Model file for the job. Use its own axes, mm. A direction names the side the tool comes from. Give positions to 0.01 mm unless a question says otherwise; leave off trailing zeros. Order: outer loops, then holes, each group sorted by start corner. A loop starts at its lowest first (then second) coordinate and runs counter-clockwise, first axis right, second up. Notation, with made-up numbers: (-23, 3.25) -> (16, 3.25) arc R26 cw to (16, 28.25) -> close; hole circle Ø8 at (65, 50.5). An arc over 180 degrees is marked (long way). Use CSV: the item, a comma, the result in double quotes. Start each with the question number.
1. Cut at D-D on x = 240.5. List the corners of the cut face in (y, z).
2. 3-axis set-ups, long thin cutter, end or side, ignore diameter. For faces 5 (the flat face through (238.6, 4.3, 3.2)), 6 (the flat face through (243, -5.677, 9)), 7 (the flat face through (241, 4, 0)): which of +Z, -Z, +X, -X, +Y, -Y reach the whole face in a straight line?
3. Cut at C-C on y = 11.5. List the corners of the cut face in (x, z).
4. Cut at B-B on z = 6.5. List the corners of the cut face in (x, y), then the cut area to 3 significant figures.
5. Drop flat-ended pins along their axis: pin 1 (4 mm diameter, centred on x = 241, z = 10.5, fed in from +Y); pin 2 (5 mm diameter, centred on y = 16.5, z = 11.5, fed in from +X); pin 3 (2 mm diameter, centred on x = 234.5, y = 2, fed in from +Z). Give the stop position or say it passes through.
6. Cut at A-A on z = 4.25. List the corners of the cut face in (x, y), then the cut area to 3 significant figures.
7. Pull direction Y, two halves, no side cores. Call faces 1 (the cylindrical face through (228.141, -4.775, 9.056)), 2 (the flat face through (239, 6, 5)), 3 (the flat face through (236, 6.073, 3)), 4 (the flat face through (236, -0.827, 3)): released by +Y, released by -Y, zero draft, split by the parting line, or undercut.
8. Wall check: line 1 (Z direction, x = 233, y = 6); line 2 (X direction, y = 3, z = 9); line 3 (Y direction, x = 239, z = 9.5). Give the ranges that are in metal, low to high. Write a range as from..to.
```python
from build123d import *

# Parameters (mm, degrees)
SKETCH1_R           = 2.1
BOSS_EXTRUDE1_DEPTH = 5
BOSS_EXTRUDE2_DEPTH = 8
FILLET1_R           = 3
CUT_EXTRUDE1_DEPTH  = 3.6
FILLET2_R           = 5
FILLET3_R           = 1


with BuildPart() as part:
    # Sketch1 → Boss-Extrude1 (new body)
    with BuildSketch(Plane.XY):
        Polygon((257.428056395, -9.677220034), (223.285920771, -9.677220034), (223.285920771, 24.46491559), (233.285920771, 24.46491559), (257.428056395, 0.322779966), align=None)
        with Locations((235.585920771, 2.622779966)):
            Circle(SKETCH1_R, mode=Mode.SUBTRACT)
    extrude(amount=BOSS_EXTRUDE1_DEPTH)

    # Sketch2 → Boss-Extrude2 (add)
    with BuildSketch(Plane.XY.offset(5)):
        Polygon((257.428056395, -9.677220034), (223.285920771, -9.677220034), (223.285920771, 24.46491559), (227.285920771, 24.46491559), (227.285920771, -5.677220034), (257.428056395, -5.677220034), align=None)
    extrude(amount=BOSS_EXTRUDE2_DEPTH)

    # Fillet1
    fillet1_edges = [part.edges().sort_by_distance(p)[0] for p in [
        (227.285920771, -5.677220034, 9),
        (223.285920771, -9.677220034, 6.5),
    ]]
    fillet(fillet1_edges, radius=FILLET1_R)

    # Sketch3 → Cut-Extrude1 (cut)
    with BuildSketch(Plane.XY.offset(5)):
        Polygon((239.569637629, 2.622779966), (237.5777792, 6.072779966), (233.594062342, 6.072779966), (231.602203914, 2.622779966), (233.594062342, -0.827220034), (237.5777792, -0.827220034), align=None)
    extrude(amount=-CUT_EXTRUDE1_DEPTH, mode=Mode.SUBTRACT)

    # Fillet2
    fillet2_edges = [part.edges().sort_by_distance(p)[0] for p in [
        (233.285920771, 24.46491559, 2.5),
        (257.428056395, 0.322779966, 2.5),
    ]]
    fillet(fillet2_edges, radius=FILLET2_R)

    # Fillet3
    fillet3_edges = [part.edges().sort_by_distance(p)[0] for p in [
        (257.428056395, -5.677220034, 9),
        (227.285920771, 24.46491559, 9),
        (257.428056395, -9.677220034, 6.5),
        (223.285920771, 24.46491559, 6.5),
    ]]
    fillet(fillet3_edges, radius=FILLET3_R)


solid = part.part
```
Verdict:
1,outline,"(-9.68, 0) -> (17.25, 0) -> (17.25, 5) -> (-5.68, 5) -> (-5.68, 13) -> (-9.68, 13) -> close"
2,face 5,"+Z"
2,face 6,"+Z, +X, +Y"
2,face 7,"-Z, +X, -X, +Y, -Y"
3,outline,"(223.29, 0) -> (246.25, 0) -> (246.25, 5) -> (227.29, 5) -> (227.29, 13) -> (223.29, 13) -> close"
4,outline,"(223.29, -6.68) arc R3 ccw to (226.29, -9.68) -> (256.43, -9.68) arc R1 ccw to (257.43, -8.68) -> (257.43, -6.68) arc R1 ccw to (256.43, -5.68) -> (230.29, -5.68) arc R3 cw to (227.29, -2.68) -> (227.29, 23.46) arc R1 ccw to (226.29, 24.46) -> (224.29, 24.46) arc R1 ccw to (223.29, 23.46) -> close"
4,area,"256 mm^2"
5,pin 1,"y = -5.68"
5,pin 2,"x = 227.29"
5,pin 3,"z = 1.4"
6,outline,"(223.29, -6.68) arc R3 ccw to (226.29, -9.68) -> (256.43, -9.68) arc R1 ccw to (257.43, -8.68) -> (257.43, -1.75) arc R5 ccw to (255.96, 1.79) -> (234.75, 23) arc R5 ccw to (231.21, 24.46) -> (224.29, 24.46) arc R1 ccw to (223.29, 23.46) -> close; hole (231.6, 2.62) -> (233.59, -0.83) -> (237.58, -0.83) -> (239.57, 2.62) -> (237.58, 6.07) -> (233.59, 6.07) -> close"
6,area,"830 mm^2"
7,face 1,"released by +Y"
7,face 2,"zero draft"
7,face 3,"undercut"
7,face 4,"undercut"
8,line 1,"0..5"
8,line 2,"223.29..227.29"
8,line 3,"-9.68..-5.68"
